Autodesk Inventor part; units mm, degrees
ref_plane "YZ Plane" through (0, 0, 0) normal (1, 0, 0) x (0, 1, 0)
ref_plane "XZ Plane" through (0, 0, 0) normal (0, 1, 0) x (-1, 0, 0)
ref_plane "XY Plane" through (0, 0, 0) normal (0, 0, 1) x (1, 0, 0)
sketch "Sketch1" plane through (0, 0, 0) normal (0, 1, 0) x (-1, 0, 0)
  line L0 (-11.5, 25) -> (11.5, 25)
  line L1 (11.5, 25) -> (11.5, -25)
  line L2 (11.5, -25) -> (-11.5, -25)
  line L3 (-11.5, -25) -> (-11.5, 25)
  line L4 (-11.5, 25) -> (11.5, -25) construction
  line L5 (11.5, 25) -> (-11.5, -25) construction
  line L6 (-13.1, -26.6) -> (13.1, -26.6)
  line L7 (13.1, -26.6) -> (13.1, 26.6)
  line L8 (13.1, 26.6) -> (-13.1, 26.6)
  line L9 (-13.1, 26.6) -> (-13.1, -26.6)
  line L10 (-13.1, -26.6) -> (13.1, 26.6) construction
  line L11 (13.1, -26.6) -> (-13.1, 26.6) construction
  point P0 (0, 0)
  dimension "d0" = 23
  dimension "d1" = 50
  dimension "d2" = 1.6
  dimension "d3" = 1.6
extrude "Extrusion1" add sketch "Sketch1" along normal blind 20
sketch "Sketch2" plane through (0, 0, 0) normal (0, -1, 0) x (1, 0, 0)
  line L0 (-11.5, -25) -> (-11.5, 25)
  line L1 (-11.5, 25) -> (11.5, 25)
  line L2 (11.5, 25) -> (11.5, -25)
  line L3 (11.5, -25) -> (-11.5, -25)
  point P0 (0, 0)
extrude "Extrusion2" add sketch "Sketch2" against normal blind 1.6
sketch "Sketch3" plane through (0, 1.6, 0) normal (0, 1, 0) x (1, 0, 0)
  line L0 (-11.5, 25) -> (11.5, 25)
  line L1 (-10.5, 9) -> (10.5, 9)
  line L2 (10.5, 9) -> (10.5, -23)
  line L3 (10.5, -23) -> (-10.5, -23)
  line L4 (-10.5, -23) -> (-10.5, 9)
  line L5 (-10.5, 9) -> (10.5, -23) construction
  line L6 (10.5, 9) -> (-10.5, -23) construction
  circle A0 centre (-7, 5.5) radius 1.3
  circle A1 centre (-7, 5.5) radius 3.5
  point P0 (0, 0)
  point P1 (0, -7)
  dimension "d8" = 21
  dimension "d9" = 32
  dimension "d10" = 16
  dimension "d11" = 2.6
  dimension "d26" = 3.5
  dimension "d27" = 3.5
  dimension "d29" = 7
extrude "Extrusion3" add sketch "Sketch3" along normal blind 4 contours A1
sketch "Sketch4" plane through (-13.1, 0, 26.6) normal (0, 0, 1) x (1, 0, 0)
  line L0 (0, 0) -> (26.2, 0)
  line L1 (1.6, 1.6) -> (1.6, 20)
  line L2 (1.6, 1.6) -> (1.6, 20)
  line L3 (24.6, 1.6) -> (24.6, 20)
  line L4 (24.6, 1.6) -> (24.6, 20)
  line L5 (1.6, 4) -> (24.1799, 4)
  line L6 (24.1799, 4) -> (24.1799, 10)
  line L7 (24.1799, 10) -> (1.6, 10)
  line L8 (1.6, 10) -> (1.6, 4)
  point P0 (13.1, 0)
  dimension "d16" = 6
  dimension "d17" = 4
extrude "Extrusion4" cut sketch "Sketch4" against normal blind 4
sketch "Sketch5" plane through (0, 1.6, 0) normal (0, 1, 0) x (1, 0, 0)
  line L0 (-11.5, -25) -> (-11.5, 25)
  line L1 (11.5, -25) -> (-11.5, -25)
  line L2 (11.5, 25) -> (11.5, -25)
  line L3 (6.8, 0) -> (8, 0)
  line L4 (8, 0) -> (8, -25)
  line L5 (8, -25) -> (6.8, -25)
  line L6 (6.8, -25) -> (6.8, 0)
  line L7 (-8, 0) -> (-6.8, 0)
  line L8 (-6.8, 0) -> (-6.8, -25)
  line L9 (-6.8, -25) -> (-8, -25)
  line L10 (-8, -25) -> (-8, 0)
  point P0 (0, 0)
  dimension "d20" = 1.2
  dimension "d21" = 1.2
  dimension "d22" = 3.5
  dimension "d23" = 3.5
extrude "Extrusion5" add sketch "Sketch5" along normal blind 4
fillet "Fillet1" radius 3 4 edges at (13.1, 10, 26.6) (13.1, 10, -26.6) (-13.1, 10, -26.6) (-13.1, 10, 26.6)
sketch "Sketch6" plane through (10.1, 0, -26.6) normal (0, 0, -1) x (-1, 0, 0)
  circle A0 centre (10.1, 10) radius 2.6
  point P0 (10.1, 0)
  dimension "d31" = 5.2
extrude "Extrusion6" cut sketch "Sketch6" against normal blind 4
sketch "Sketch7" plane through (10.1, 0, -26.6) normal (0, 0, -1) x (-1, 0, 0)
  circle A0 centre (10.1, 10) radius 2.6
  circle A1 centre (10.1, 10) radius 4
  point P0 (10.1, 0)
  dimension "d34" = 8
extrude "Extrusion7" add sketch "Sketch7" along normal blind 2
fillet "Fillet2" radius 3 2 edges at (4, 10, -26.6) (4, 10, -28.6)
sketch "Sketch8" plane through (-11.5, 20, 25) normal (1, 0, 0) x (0, 0, -1)
  line L0 (-1.2533, -16) -> (-1.2533, -10)
  line L1 (-1.2533, -16) -> (0, -16)
  line L2 (0, -18.4) -> (0, -16)
  line L3 (0, -18.4) -> (50, -18.4)
  line L4 (50, -18.4) -> (50, 0)
  line L5 (0, 0) -> (50, 0)
  line L6 (0, -10) -> (0, 0)
  line L7 (-1.2533, -10) -> (0, -10)
  line L8 (27, -18.4) -> (34, -18.4)
  line L9 (29.2, -14.4) -> (31.8, -14.4)
  line L10 (34, -14.4) -> (27, -14.4)
  point P0 (25, -20)
  dimension "d38" = 14.4
sketch "Sketch9" plane through (11.5, 20, 25) normal (0, 0, -1) x (-1, 0, 0)
  line L0 (23, -10) -> (23, 0)
  line L1 (0, 0) -> (23, 0)
  line L2 (23, 0) -> (23, -1.4)
  line L3 (23, -1.4) -> (0, -1.4)
  line L4 (0, -1.4) -> (0, 0)
  point P0 (11.5, -20)
  dimension "d39" = 1.4
extrude "Extrusion8" add sketch "Sketch9" along normal blind 2
sketch "Sketch10" plane through (0, 1.6, 0) normal (0, 1, 0) x (1, 0, 0)
  line L0 (11.5, 25) -> (11.5, -25)
  line L1 (-11.5, 25) -> (11.5, 25)
  line L2 (-11.5, -25) -> (-11.5, 25)
  circle A0 centre (-8.3566, 21.8566) radius 1.2
  circle A1 centre (-8.3566, 21.8566) radius 3.1434
  circle A2 centre (8.3566, 21.8566) radius 1.2
  circle A3 centre (8.3566, 21.8566) radius 3.1434
  point P0 (0, 0)
  dimension "d45" = 2.4
  dimension "d46" = 3.1434
  dimension "d47" = 3.1434
  dimension "d48" = 2.4
  dimension "d49" = 3.1434
  dimension "d50" = 3.1434
extrude "Extrusion9" add sketch "Sketch10" along normal up to surface (18.4 mm away) contours A3 | A1
chamfer "Chamfer2" distance 1 angle 45 1 edges at (0, 18.6, 23)
sketch "Sketch11" plane through (0, 1.6, 0) normal (0, 1, 0) x (1, 0, 0)
  circle A0 centre (0, 15.6096) radius 1.7
  point P0 (0, 0)
  dimension "d56" = 3.4
extrude "Extrusion10" cut sketch "Sketch11" against normal through all
equation "\"d3\" = d2"
equation "\"d47\" = d46"
equation "\"d49\" = d47"
equation "\"d50\" = d46"
properties part number "bottom v3"
Model file for the job. Use its own axes, mm. A direction names the side the tool comes from. Round coordinates to 2 decimals unless told otherwise and drop trailing zeros. Order: outer loops, then holes, each group sorted by start corner. A loop starts at its lowest first (then second) coordinate and runs counter-clockwise, first axis right, second up.
(1) Band-saw the part on B-B (x = 0). Give the number of separate pieces and of enclosed holes in the cut face, then the cut area to 3 significant figures.
(2) Pin check, flat tips, straight feed: pin 1 (1.9 mm diameter, centred on x = 8.36, z = -21.86, fed in from +Y); pin 2 (1.6 mm diameter, centred on y = 7, z = 26, fed in from -X); pin 3 (1.5 mm diameter, centred on x = -0.5, y = 9.5, fed in from -Z). Stop position of each tip, or through.
(3) 3-axis set-ups, long thin cutter, end or side, ignore diameter. For faces 1 (the face through (0.2, 19.1, 23.5)), 2 (the face through (-7, 1.6, -5)), 3 (the face through (13.1, 10, 0)), 4 (the face through (7, 10, -26.6)): which of +Z, -Z, +X, -X, +Y, -Y reach the whole face in a straight line?
(4) Band-saw the part on C-C (z = -5.5). List the corners of the cut face in (x, y), then the cut area to 3 significant figures.
(5) Pull direction X, two halves, no side cores. Call faces 5 (the face through (-10.497, 3.572, -5.346)), 6 (the face through (-12.2, 9.86, 25.74)), 7 (the face through (0, 15, 26.6)): released by +X, released by -X, zero draft, split by the parting line, or undercut.
(6) Band-saw the part on A-A (z = 2). List the corners of the cut face in (x, y), then the cut area to 3 significant figures.
(7) Drill centre lines: line 1 (X direction, y = 16.5, z = -10); line 2 (Z direction, x = 5.5, y = 17); line 3 (Z direction, x = -10.75, y = 10.5). Where is each one in solid material? Low to high.
Verdict:
1. separate pieces: 4
1. enclosed holes: 0
1. area: 131 mm2
2. pin 1: stops at y = 1.6
2. pin 2: stops at x = -12.64
2. pin 3: stops at z = 25
3. face 1: none
3. face 2: +Y
3. face 3: +Z, -Z, +X, +Y, -Y
3. face 4: -Z
4. outline: (-13.1, 0) - (13.1, 0) - (13.1, 20) - (11.5, 20) - (11.5, 1.6) - (-3.5, 1.6) - (-3.5, 5.6) - (-5.7, 5.6) - (-5.7, 1.6) - (-8.3, 1.6) - (-8.3, 5.6) - (-10.5, 5.6) - (-10.5, 1.6) - (-11.5, 1.6) - (-11.5, 20) - (-13.1, 20) - close
4. area: 118 mm2
5. face 5: undercut
5. face 6: released by -X
5. face 7: zero draft
6. outline: (-13.1, 0) - (13.1, 0) - (13.1, 20) - (11.5, 20) - (11.5, 1.6) - (8, 1.6) - (8, 5.6) - (6.8, 5.6) - (6.8, 1.6) - (-6.8, 1.6) - (-6.8, 5.6) - (-8, 5.6) - (-8, 1.6) - (-11.5, 1.6) - (-11.5, 20) - (-13.1, 20) - close
6. area: 110 mm2
7. line 1: x = -13.1 to -11.5, 11.5 to 13.1
7. line 2: z = -26.6 to -25, -23.17 to -20.54, 25 to 26.6
7. line 3: z = -26.53 to -25, -23.89 to -19.82, 25 to 26.53
